Design review of the part shown in the three views and the two pictorial views. Dimensions are in mm from the part's minimum x, y and z. Round coordinates to 2 decimals unless told otherwise and drop trailing zeros. Write each loop counter-clockwise with the first axis right and the second up, starting at its lowest first coordinate (ties: lowest second). Pieces come first, ordered by that corner, then holes. Notation, with made-up numbers: (-19.75, 59) - (25.25, 59) arc R17 cw to (25.25, 77) - close; hole circle Ø6 at (-30, -24.75). An arc over 180 degrees is marked (long way). Use one line per item in the form item = value.
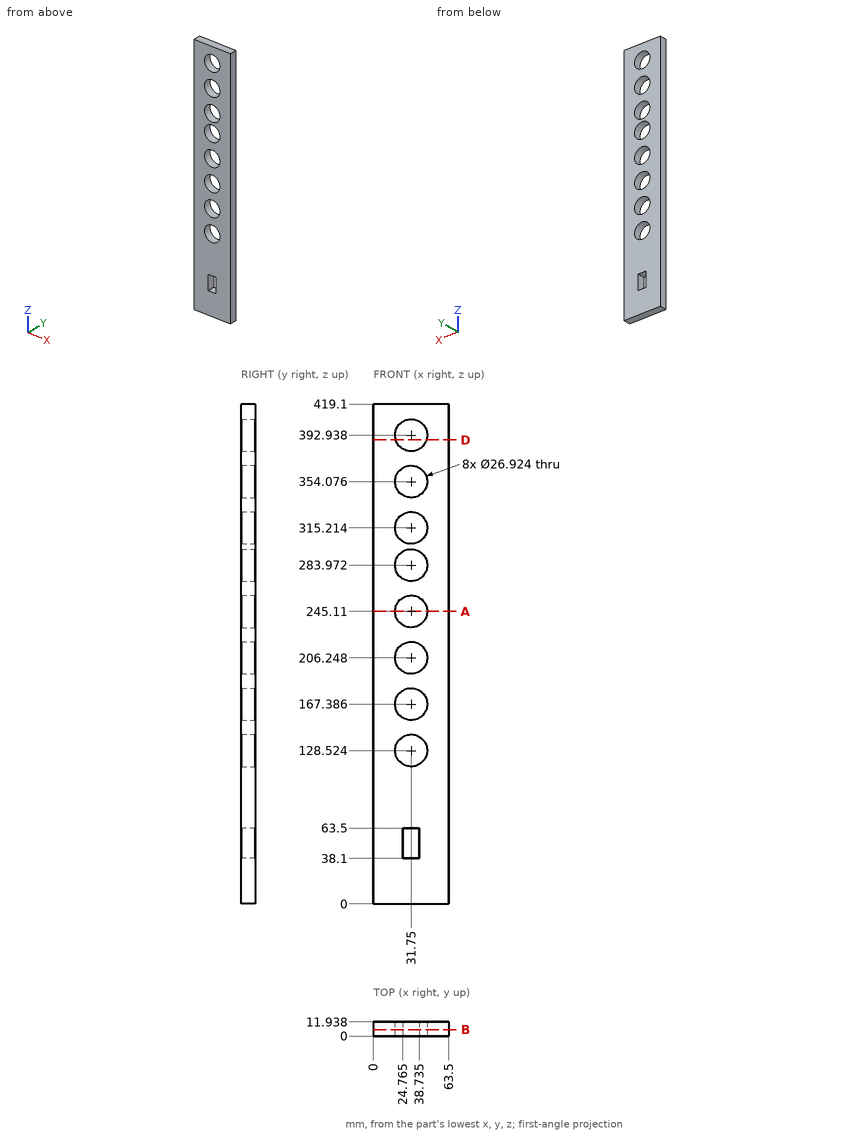
(1) Insertion check: P1, Ø12, axis at x = 35, z = 99.5, coming from the -Y side. The pin has a flat end and moves straight along its axis. Give the tip position at first contact, or say it passes through.
Geometry results:
P1 = 0
(2) Add section B-B on y = 5.25. Count the separate pieces of the cut face and the enclosed holes in it, then the cut area to 3 significant figures.
Geometry results:
separate_pieces = 1
enclosed_holes = 9
area = 21,700 mm2
(3) To check wall thickness, follow L1, parallel to X at y = 7, z = 167; L2, parallel to X at y = 3, z = 59.5 (3 decimals). State the ranges of each line that lie inside material, in increasing order.
Geometry results:
L1 = 0 to 18.29, 45.21 to 63.5
L2 = 0 to 24.765, 38.735 to 63.5
(4) Add section A-A on z = 245.11. Write out the cut boundary in (x, y), then the cut area to 3 significant figures.
Geometry results:
outline = (0, 0) - (18.29, 0) - (18.29, 11.94) - (0, 11.94) - close; (45.21, 0) - (63.5, 0) - (63.5, 11.94) - (45.21, 11.94) - close
area = 437 mm2
(5) Add section D-D on z = 389. Write out the cut boundary in (x, y), then the cut area to 3 significant figures.
Geometry results:
outline = (0, 0) - (18.88, 0) - (18.88, 11.94) - (0, 11.94) - close; (44.62, 0) - (63.5, 0) - (63.5, 11.94) - (44.62, 11.94) - close
area = 451 mm2
